from build123d import *

# Parameters (mm, degrees)
BOSS_EXTRUDE1_DEPTH = 53
SKETCH2_W           = 2.4
SKETCH2_H           = 4
CUT_EXTRUDE1_DEPTH  = 0.3
SKETCH3_W           = 4
SKETCH3_H           = 4
CUT_EXTRUDE2_DEPTH  = 2.5


with BuildPart() as part:
    # Sketch1 → Boss-Extrude1 (new body)
    with BuildSketch(Plane.XY):
        with BuildLine():
            Line((-14, 3), (14, 3))
            ThreePointArc((14, 3), (17, 0), (14, -3))
            Line((14, -3), (-14, -3))
            ThreePointArc((-14, -3), (-17, 0), (-14, 3))
        make_face()
    extrude(amount=BOSS_EXTRUDE1_DEPTH)

    # Sketch2 → Cut-Extrude1 (cut)
    with BuildSketch(Plane.XY.offset(53)):
        with Locations((-12.5, 0)):
            Rectangle(SKETCH2_W, SKETCH2_H)
        with Locations((-9.5, 0)):
            Rectangle(SKETCH2_W, SKETCH2_H)
        with Locations((-6.5, 0)):
            Rectangle(SKETCH2_W, SKETCH2_H)
    extrude(amount=-CUT_EXTRUDE1_DEPTH, mode=Mode.SUBTRACT)

    # Sketch3 → Cut-Extrude2 (cut)
    with BuildSketch(Plane.XY.offset(53)):
        with Locations((-17.1, -2)):
            Rectangle(SKETCH3_W, SKETCH3_H)
        with Locations((17.1, -2)):
            Rectangle(SKETCH3_W, SKETCH3_H)
    extrude(amount=-CUT_EXTRUDE2_DEPTH, mode=Mode.SUBTRACT)


solid = part.part
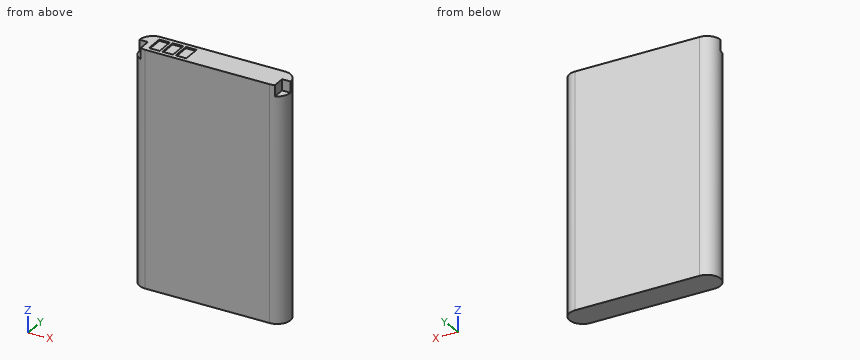
Work out the finished part from the listing and answer in its coordinate system (mm). Round coordinates to 2 decimals unless told otherwise and drop trailing zeros. Write each loop counter-clockwise with the first axis right and the second up, starting at its lowest first coordinate (ties: lowest second). Pieces come first, ordered by that corner, then holes.
1) A cutting plane is placed at A-A (z = 18.5). Give the vertices of the cut face in (x, y).
2) Straight lines are drawn through the part: line 1 (Z direction, x = -11.5, y = 1.25); line 2 (X direction, y = 0.2, z = 27.5); line 3 (X direction, y = 1.2, z = 6). For each, find the intervals that lie inside material, in ascending order.
3) Given pin 1 Ø2 at (y, z) = (-1.5, 52) entering from -X; pin 2 Ø1 at (x, y) = (-16.5, -1) entering from +Z; pin 3 Ø2 at (x, z) = (16, 51.5) entering from -Y, each flat-ended and moving along its own axis, determine where each tip first touches the part or whether it passes through.
Completed:
1. outline: (-14, -3) - (14, -3) arc R3 ccw to (14, 3) - (-14, 3) arc R3 ccw to start
2. line 1: z = 0 to 52.7
2. line 2: x = -16.99 to 16.99
2. line 3: x = -16.75 to 16.75
3. pin 1: stops at x = -15.1
3. pin 2: stops at z = 50.5
3. pin 3: stops at y = -2.83
